from build123d import *

# Parameters (mm, degrees)
SKETCH1_R           = 16.5
BOSS_EXTRUDE1_DEPTH = 19.5
SHELL1_T            = -0.5
SKETCH2_R           = 3
CUT_EXTRUDE1_DEPTH  = 31.409702399
FILLET1_R           = 0.5


with BuildPart() as part:
    # Sketch1 → Boss-Extrude1 (new body)
    with BuildSketch(Plane.XY):
        Circle(SKETCH1_R)
    extrude(amount=-BOSS_EXTRUDE1_DEPTH)

    # Shell1
    shell1_openings = [part.faces().sort_by_distance(p)[0] for p in [
        (0, 0, -19.5),
    ]]
    offset(amount=SHELL1_T, openings=shell1_openings, kind=Kind.INTERSECTION)

    # Sketch2 → Cut-Extrude1 (cut, through all)
    with BuildSketch(Plane.XY):
        Circle(SKETCH2_R)
    extrude(amount=-CUT_EXTRUDE1_DEPTH, mode=Mode.SUBTRACT)

    # Fillet1
    fillet1_edges = [part.edges().sort_by_distance(p)[0] for p in [
        (-16.5, 0, 0),
    ]]
    fillet(fillet1_edges, radius=FILLET1_R)


solid = part.part
Build history of the part. All positions in model axes, mm. A direction names the side the tool comes from. Round coordinates to 2 decimals unless told otherwise and drop trailing zeros. Loops run counter-clockwise (first coordinate to the right, second up) from the corner with the lowest first, then second, coordinate; pieces in that order, holes last. Notation, with made-up numbers: (-8, -7) -> (13, -7) arc R20 ccw to (13, 0) -> close; hole circle Ø6 at (25, 46.5). An arc over 180 degrees is marked (long way). Use CSV: the item, a comma, the result in double quotes. Start each with the question number.
Q1. Saw through at A-A on x = 0. Give the cut face in (y, z), and give its area (3 significant figures).
Q2. Drill centre lines: L1, parallel to Y at x = 0, z = -12; L2, parallel to Z at x = -5, y = -9.5; L3, parallel to Y at x = -2, z = -4.75. Where is each one in solid material? Low to high.
Q3. Saw through at C-C on z = -9. Give the cut face in (x, y).
Q4. Flat gauge pins, fed straight in: pin 1 Ø5 at (y, z) = (11, -12) entering from -X; pin 2 Ø1.5 at (x, z) = (-7.5, -8) entering from +Y; pin 3 Ø3 at (y, z) = (-6.5, -13) entering from -X. Where does each tip first touch, or does it go through?
Q5. Which spindle directions (+Z, -Z, +X, -X, +Y, -Y) get a long thin tool onto all of the face, cutting with end or side? Do faces 4 (the face through (3.3, 0.2, 0)), 5 (the face through (-3.47, -15.62, -9.87)). Say none if no direction does.
Q6. Mould opens along X. For faces 1 (the face through (3.3, 0.2, -0.5)), 2 (the face through (-16, 3, -19.5)), 3 (the face through (15.24, -6.32, -9.87)) say: +X half, -X half, draft (parallel to the pull), parting line (faces both ways), or undercut.
Solutions:
1,outline,"(-16.5, -19.5) -> (-16, -19.5) -> (-16, -0.5) -> (-3, -0.5) -> (-3, 0) -> (-16, 0) arc R0.5 ccw to (-16.5, -0.5) -> close; (3, -0.5) -> (16, -0.5) -> (16, -19.5) -> (16.5, -19.5) -> (16.5, -0.5) arc R0.5 ccw to (16, 0) -> (3, 0) -> close"
1,area,"32.4 mm^2"
2,L1,"y = -16.5 to -16, 16 to 16.5"
2,L2,"z = -0.5 to 0"
2,L3,"y = -16.38 to -15.87, 15.87 to 16.38"
3,outline,"circle Ø33 at (0, 0); hole circle Ø32 at (0, 0)"
4,pin 1,"stops at x = -14.14"
4,pin 2,"stops at y = 15.06"
4,pin 3,"stops at x = -15.72"
5,face 4,"+Z, +X, -X, +Y, -Y"
5,face 5,"-Z"
6,face 1,"undercut"
6,face 2,"draft"
6,face 3,"parting line"
